from build123d import *

# Parameters (mm, degrees)
SKETCH1_R           = 17
BOSS_EXTRUDE1_DEPTH = 30
SKETCH2_R           = 16
CUT_EXTRUDE1_DEPTH  = 3
SKETCH3_R           = 1
CUT_EXTRUDE2_DEPTH  = 2
FILLET1_R           = 1


with BuildPart() as part:
    # Sketch1 → Boss-Extrude1 (new body)
    with BuildSketch(Plane(origin=(0, 0, 0), x_dir=(1, 0, 0), z_dir=(0, 1, 0))):
        Circle(SKETCH1_R)
    extrude(amount=BOSS_EXTRUDE1_DEPTH)

    # Sketch2 → Cut-Extrude1 (cut)
    with BuildSketch(Plane(origin=(0, 30, 0), x_dir=(1, 0, 0), z_dir=(0, 1, 0))):
        Circle(SKETCH2_R)
    extrude(amount=-CUT_EXTRUDE1_DEPTH, mode=Mode.SUBTRACT)

    # Sketch3 → Cut-Extrude2 (cut)
    with BuildSketch(Plane.XZ):
        Circle(SKETCH3_R)
    extrude(amount=-CUT_EXTRUDE2_DEPTH, mode=Mode.SUBTRACT)

    # Fillet1
    fillet1_edges = [part.edges().sort_by_distance(p)[0] for p in [
        (-1, 2, 0),
    ]]
    fillet(fillet1_edges, radius=FILLET1_R)


solid = part.part
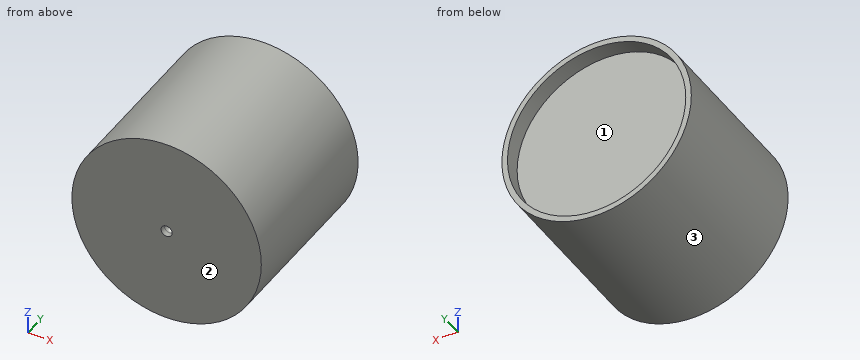
Input: part model. Units: mm. Frame: model coordinates. Face numbers are marked on the shaded views. Round coordinates to 2 decimals unless told otherwise and drop trailing zeros. Order: outer loops, then holes, each group sorted by start corner. A loop starts at its lowest first (then second) coordinate and runs counter-clockwise, first axis right, second up. Notation, with made-up numbers: (88.25, 42) - (128.25, 42) arc R25 cw to (128.25, 72) - close; hole circle Ø2 at (54, 61.5). An arc over 180 degrees is marked (long way). Use a Markdown table: item, result.
1. Section A-A on x = 0. Return the cut outline in (y, z).
Evaluation:
| item | result |
|---|---|
| outline | (0, -17) - (30, -17) - (30, -16) - (27, -16) - (27, 16) - (30, 16) - (30, 17) - (0, 17) - (0, 1) - (1, 1) arc R1 cw to (1, -1) - (0, -1) - close |
2. Mould query, pull axis Z, two halves, no side actions, for the marked faces 1, 2 and 3. Classes: +Z half, -Z half, draft (parallel to the pull), parting line (faces both ways), or undercut.
Evaluation:
| item | result |
|---|---|
| face 1 | undercut |
| face 2 | draft |
| face 3 | parting line |
3. First-contact query: pin 1 (19 mm diameter, centred on x = 0, z = 0, fed in from -Y); pin 2 (10 mm diameter, centred on y = 20.5, z = 9, fed in from -X); pin 3 (6 mm diameter, centred on x = -6, y = 18.5, fed in from +Z); pin 4 (1 mm diameter, centred on y = 21.5, z = -10.5, fed in from -X). Flat tips, straight axial feed; report the tip coordinate or a pass-through.
Evaluation:
| item | result |
|---|---|
| pin 1 | y = 0 |
| pin 2 | x = -16.52 |
| pin 3 | z = 16.73 |
| pin 4 | x = -13.75 |
4. Section D-D on x = -4. Return the cut outline in (y, z).
Evaluation:
| item | result |
|---|---|
| outline | (0, -16.52) - (30, -16.52) - (30, -15.49) - (27, -15.49) - (27, 15.49) - (30, 15.49) - (30, 16.52) - (0, 16.52) - close |
5. Material intervals for probe 1 along Z at (x, y) = (0, 0.6); probe 2 along X at (y, z) = (29.1, 0), sorted ascending.
Evaluation:
| item | result |
|---|---|
| probe 1 | -17 to -1, 1 to 17 |
| probe 2 | -17 to -16, 16 to 17 |
6. Section C-C on y = 13. Return the cut outline in (x, z), then the cut area to 3 significant figures.
Evaluation:
| item | result |
|---|---|
| outline | circle Ø34 at (0, 0) |
| area | 908 mm^2 |
7. Section B-B on z = 0. Return the cut outline in (x, y).
Evaluation:
| item | result |
|---|---|
| outline | (-17, 0) - (-1, 0) - (-1, 1) arc R1 cw to (1, 1) - (1, 0) - (17, 0) - (17, 30) - (16, 30) - (16, 27) - (-16, 27) - (-16, 30) - (-17, 30) - close |
